from build123d import *

# Parameters (mm, degrees)
F0_R     = 4.826
F1_DEPTH = 127
F0_W     = 5.08
F0_H     = 3.3782
F2_DEPTH = 3.81
F3_DEPTH = 25.4
F4_R     = 4.826
F5_DEPTH = 6.35


with BuildPart() as f1:
    # F0 (on Top) → F1 (new body)
    with BuildSketch(Plane.XY):
        with BuildLine():
            ThreePointArc((-2.54, 7.184205), (-4.399409, -6.221704), (7.62, 0))
            ThreePointArc((7.62, 0), (6.221704, 4.399409), (2.54, 7.184205))
            ThreePointArc((2.54, 7.184205), (0, 7.62), (-2.54, 7.184205))
        make_face()
        Circle(F0_R, mode=Mode.SUBTRACT)
    extrude(amount=-F1_DEPTH)

    # F0 (on Top) → F2 (join)
    with BuildSketch(Plane.XY):
        with BuildLine():
            ThreePointArc((-2.54, 7.184205), (-4.399409, -6.221704), (7.62, 0))
            ThreePointArc((7.62, 0), (6.221704, 4.399409), (2.54, 7.184205))
            ThreePointArc((2.54, 7.184205), (0, 7.62), (-2.54, 7.184205))
        make_face()
        Circle(F0_R, mode=Mode.SUBTRACT)
        with BuildLine():
            ThreePointArc((-2.54, 7.184205), (0, 7.62), (2.54, 7.184205))
            Line((2.54, 7.184205), (2.54, 10.156005))
            Line((2.54, 10.156005), (-2.54, 10.156005))
            Line((-2.54, 10.156005), (-2.54, 7.184205))
        make_face()
        with Locations((0, 11.845105)):
            Rectangle(F0_W, F0_H)
    extrude(amount=F2_DEPTH)

    # F0 (on Top) → F3 (join)
    with BuildSketch(Plane.XY):
        with Locations((0, 11.845105)):
            Rectangle(F0_W, F0_H)
    extrude(amount=-F3_DEPTH)

    # F4 (on face) → F5 (join)
    with BuildSketch(Plane(origin=(0, 0, -127), x_dir=(1, 0, 0), z_dir=(0, 0, -1))):
        Circle(F4_R)
    extrude(amount=-F5_DEPTH)


solid = f1.part
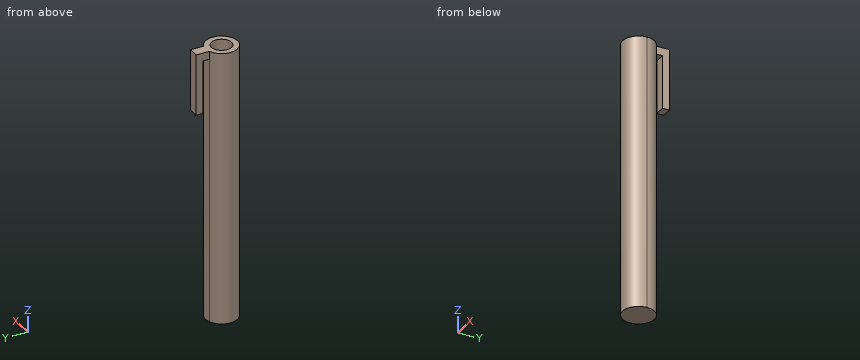
CAD build for the part. Positions are in the model's coordinates, mm. Coordinates: 2 decimals unless noted, no trailing zeros. Write each loop counter-clockwise with the first axis right and the second up, starting at its lowest first coordinate (ties: lowest second). Pieces come first, ordered by that corner, then holes. Notation, with made-up numbers: (53, 56.5) - (85, 56.5) arc R16 ccw to (85, 82.5) - close; hole circle Ø3 at (63.5, 20). An arc over 180 degrees is marked (long way). Use a Markdown table: item, result. Add a question column.
Item 1: Band-saw the part on A-A, the plane z = -15.5. Give the cut face in (x, y).
Item 2: Band-saw the part on C-C, the plane z = -49. Give the cut face in (x, y), and give its area (3 significant figures).
Item 3: Drill centre lines: L1, parallel to Y at x = 0, z = -90.5; L2, parallel to Z at x = -2.5, y = 2.25; L3, parallel to Z at x = 2.5, y = 12.75. Where is each one in solid material? Low to high. Write a range as from..to.
Item 4: Band-saw the part on B-B, the plane x = 0. Give the cut face in (y, z), and give its area (3 significant figures).
Item 5: Band-saw the part on D-D, the plane y = 3.25. Give the cut face in (x, z), and give its area (3 significant figures).
Item 6: Flat gauge pins, fed straight in: pin 1 (1.5 mm diameter, centred on x = -2.5, z = -22.5, fed in from -Y); pin 2 (1 mm diameter, centred on x = -1, y = 12.5, fed in from -Z); pin 3 (7 mm diameter, centred on y = 11, z = -9, fed in from +X); pin 4 (2.5 mm diameter, centred on x = 1, y = 8, fed in from -Z). Where does each tip first touch, or does it go through?
Numbers:
| question | item | result |
|---|---|---|
| 1 | outline | (-2.54, 7.18) arc R7.62 ccw (long way) to (2.54, 7.18) arc R7.62 ccw to start; (-2.54, 10.16) - (2.54, 10.16) - (2.54, 13.53) - (-2.54, 13.53) - close; hole circle Ø9.65 at (0, 0) |
| 2 | outline | (-2.54, 7.18) arc R7.62 ccw (long way) to (2.54, 7.18) arc R7.62 ccw to start; hole circle Ø9.65 at (0, 0) |
| 2 | area | 109 mm2 |
| 3 | L1 | -7.62..-4.83, 4.83..7.62 |
| 3 | L2 | -127..-120.65 |
| 3 | L3 | -25.4..3.81 |
| 4 | outline | (-7.62, -127) - (7.62, -127) - (7.62, 0) - (10.16, 0) - (10.16, -25.4) - (13.53, -25.4) - (13.53, 3.81) - (4.83, 3.81) - (4.83, -120.65) - (-4.83, -120.65) - (-4.83, 3.81) - (-7.62, 3.81) - close |
| 4 | area | 901 mm2 |
| 5 | outline | (-6.89, -127) - (6.89, -127) - (6.89, 3.81) - (3.57, 3.81) - (3.57, -120.65) - (-3.57, -120.65) - (-3.57, 3.81) - (-6.89, 3.81) - close |
| 5 | area | 915 mm2 |
| 6 | pin 1 | y = -7.42 |
| 6 | pin 2 | z = -25.4 |
| 6 | pin 3 | x = 2.54 |
| 6 | pin 4 | z = -127 |
